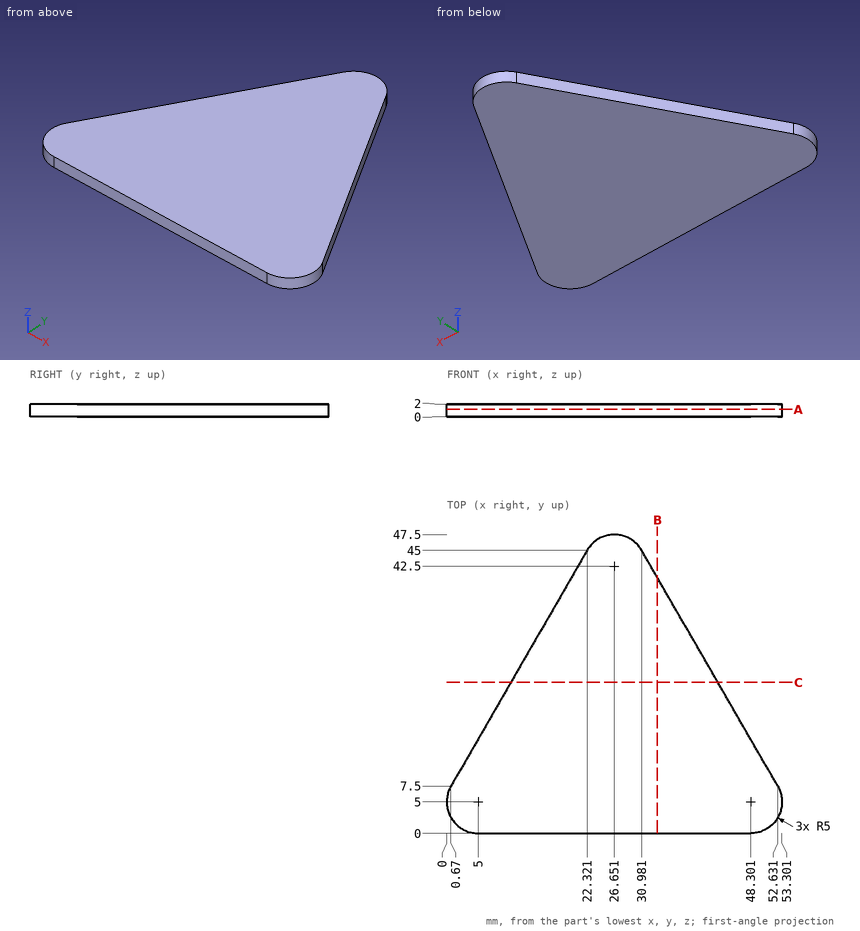
Input: dimensioned drawing with shaded views. Units: mm. Origin: part minimum x, y, z. Coordinates: 2 decimals unless noted, no trailing zeros. Loops run counter-clockwise (first coordinate to the right, second up) from the corner with the lowest first, then second, coordinate; pieces in that order, holes last. Notation, with made-up numbers: M 24,75.5 L 67,75.5 A31 ccw 67,111.5 Z; hole C 89.5,74 d6. An arc over 180 degrees is marked long. Use a Markdown table: item, result. Add a question column.
Q1. Section query C-C, the plane y = 24. Return loops of the section in (x, z) (1 decimal).
Q2. Material intervals for L1, parallel to X at y = 11, z = 0.45; L2, parallel to Y at x = 14, z = 0.5 (1 decimal); L3, parallel to Y at x = 38, z = 1.7 (1 decimal), sorted ascending.
Q3. Section query A-A, the plane z = 1.15. Return loops of the section in (x, y), and give its area (3 significant figures).
Q4. Section query B-B, the plane x = 33.5. Return loops of the section in (y, z).
Result:
| question | item | result |
|---|---|---|
| 1 | outline | M 10.2,0 L 43.1,0 L 43.1,2 L 10.2,2 Z |
| 2 | L1 | x = 2.69 to 50.61 |
| 2 | L2 | y = 0 to 30.6 |
| 2 | L3 | y = 0 to 32.8 |
| 3 | outline | M 0.67,7.5 A5 ccw 5,0 L 48.3,0 A5 ccw 52.63,7.5 L 30.98,45 A5 ccw 22.32,45 Z |
| 3 | area | 1,540 mm2 |
| 4 | outline | M 0,0 L 40.64,0 L 40.64,2 L 0,2 Z |
